Here's how the part is built. I have some questions about the finished solid (model axes, mm). A direction names the side the tool comes from. Round coordinates to 2 decimals unless told otherwise and drop trailing zeros. Write each loop counter-clockwise with the first axis right and the second up, starting at its lowest first coordinate (ties: lowest second). Pieces come first, ordered by that corner, then holes. Notation, with made-up numbers: (-39, 66.25) -> (13, 66.25) arc R19 ccw to (13, 99.25) -> close; hole circle Ø1 at (65, -1). An arc over 180 degrees is marked (long way). Put each result on its own line as item: value. Start each with the question number.
1. I need wall thicknesses on probe 1 along Z at (x, y) = (-10, -12); probe 2 along X at (y, z) = (-15, 22); probe 3 along X at (y, z) = (-8.5, -10.5). Which ranges of each line are inside material? Lowest first, please. Write a range as from..to.
2. Which directions (+Z, -Z, +X, -X, +Y, -Y) give clear straight access to the entire face, cutting with the end or side of a thin tool? Please do faces 4 (the face through (81.15, -2, 0)), 5 (the face through (72.57, -15.52, 16.15)), 6 (the face through (48, -17, 0)).
3. We'd pull the mould along Z, two halves only. Please class faces 1 (the face through (0.106, 2.465, -18.398)), 2 (the face through (105, -12, 0)), 3 (the face through (47.474, -15.521, 15.891)): +Z half, -Z half, draft (parallel to the pull), parting line (faces both ways), or undercut.
4. Suppose I cut it at A-A (z = 0). Count the separate pieces of the cut face and the enclosed holes in it, then the cut area to 3 significant figures.
5. Suppose I cut it at C-C (x = 0). Please give me the cut outline in (y, z).
6. For pin 1 (7 mm diameter, centred on x = 62, y = -5.5, fed in from +Z); pin 2 (4 mm diameter, centred on y = 0.5, z = -6, fed in from +X); pin 3 (5 mm diameter, centred on x = 74.5, z = -15.5, fed in from -Y); pin 4 (5 mm diameter, centred on x = 20.86, z = -20.86, fed in from +Y), each with a flat end and sliding along its axis, tell me the tip position at first contact or that it passes through.
7. Suppose I cut it at D-D (x = 75.5). Please give me the cut outline in (y, z).
```python
from build123d import *

# Parameters (mm, degrees)
SKETCH_1_R                   = 38
SKETCH_1_R_2                 = 12
SKETCH_1_R_3                 = 2.4
SKETCH_1_R_4                 = 3.1
EXTRUDE_1_DEPTH              = 5
SKETCH_2_R                   = 8.5
EXTRUDE_2_DEPTH              = 17
SKETCH_3_R                   = 6
CUT_EXTRUDE_1_DEPTH          = 19
CUT_EXTRUDE_2_REACH          = 59
SKETCH_4_R                   = 3.1
CUT_EXTRUDE_START            = 6
CUT_EXTRUDE_3_DEPTH          = 6
EXTRUDE_START                = -22
EXTRUDE_5_DEPTH              = 22
SKETCH_9_W                   = 41.71930009
SKETCH_9_H                   = 2.5
EXTRUDE_6_DEPTH              = 17
CUT_EXTRUDE_4_REACH          = 122.848
SKETCH_10_W                  = 15
SKETCH_10_H                  = 11
SKETCH_11_W                  = 42.3
SKETCH_11_H                  = 42.3
SKETCH_11_R                  = 11.25
CUT_EXTRUDE_5_DEPTH          = 14
CUT_EXTRUDE_6_REACH          = 113.225
SKETCH_11_2_R                = 1.75
SKETCH_11_2_R_2              = 11.25
CHAMFER_2_SIZE               = 4
HOLE_WIZARD_M5_2_D           = 5.5
HOLE_WIZARD_M5_2_CBORE_D     = 11
HOLE_WIZARD_M5_2_CBORE_DEPTH = 0.5
SKETCH_13_R                  = 3
CUT_EXTRUDE_7_DEPTH          = 3


# Read off the part's stored shape, not the designer's step: 凸台-拉伸5
with BuildPart() as part:
    # 草图1 → 凸台-拉伸1 (new body)
    with BuildSketch(Plane(origin=(0, 0, 0), x_dir=(1, 0, 0), z_dir=(0, 1, 0))):
        with Locations(Location((0, 0, 0), (0, 0, 270))):
            Circle(SKETCH_1_R)
        with Locations(Location((0, 0, 0), (0, 0, 270))):
            Circle(SKETCH_1_R_2, mode=Mode.SUBTRACT)
        with Locations(Location((-11.313708499, 11.313708499, 0), (0, 0, 270))):
            Circle(SKETCH_1_R_3, mode=Mode.SUBTRACT)
        with Locations(Location((0, 16, 0), (0, 0, 270))):
            Circle(SKETCH_1_R_3, mode=Mode.SUBTRACT)
        with Locations(Location((11.313708499, 11.313708499, 0), (0, 0, 270))):
            Circle(SKETCH_1_R_3, mode=Mode.SUBTRACT)
        with Locations(Location((11.313708499, -11.313708499, 0), (0, 0, 90))):
            Circle(SKETCH_1_R_3, mode=Mode.SUBTRACT)
        with Locations(Location((-11.313708499, -11.313708499, 0), (0, 0, 90))):
            Circle(SKETCH_1_R_3, mode=Mode.SUBTRACT)
        with Locations(Location((0, -16, 0), (0, 0, 90))):
            Circle(SKETCH_1_R_3, mode=Mode.SUBTRACT)
        with Locations(Location((-20.859650045, 20.859650045, 0), (0, 0, 270))):
            Circle(SKETCH_1_R_4, mode=Mode.SUBTRACT)
        with Locations(Location((20.859650045, 20.859650045, 0), (0, 0, 270))):
            Circle(SKETCH_1_R_4, mode=Mode.SUBTRACT)
        with Locations(Location((20.859650045, -20.859650045, 0), (0, 0, 270))):
            Circle(SKETCH_1_R_4, mode=Mode.SUBTRACT)
        with Locations(Location((-20.859650045, -20.859650045, 0), (0, 0, 270))):
            Circle(SKETCH_1_R_4, mode=Mode.SUBTRACT)
    extrude(amount=EXTRUDE_1_DEPTH)

    # 草图2 → 凸台-拉伸2 (add)
    with BuildSketch(Plane(origin=(0, 0, 0), x_dir=(1, 0, 0), z_dir=(0, 1, 0))):
        with Locations(Location((-20.859650045, 20.859650045, 0), (0, 0, 270))):
            Circle(SKETCH_2_R)
        with Locations(Location((20.859650045, 20.859650045, 0), (0, 0, 270))):
            Circle(SKETCH_2_R)
        with Locations(Location((20.859650045, -20.859650045, 0), (0, 0, 270))):
            Circle(SKETCH_2_R)
        with Locations(Location((-20.859650045, -20.859650045, 0), (0, 0, 270))):
            Circle(SKETCH_2_R)
    extrude(amount=-EXTRUDE_2_DEPTH)

    # 草图3 → 切除-拉伸1 (cut)
    with BuildSketch(Plane(origin=(0, 5, 0), x_dir=(1, 0, 0), z_dir=(0, 1, 0))):
        with Locations(Location((-20.859650045, 20.859650045, 0), (0, 0, 270))):
            Circle(SKETCH_3_R)
        with Locations(Location((20.859650045, 20.859650045, 0), (0, 0, 270))):
            Circle(SKETCH_3_R)
        with Locations(Location((20.859650045, -20.859650045, 0), (0, 0, 270))):
            Circle(SKETCH_3_R)
        with Locations(Location((-20.859650045, -20.859650045, 0), (0, 0, 270))):
            Circle(SKETCH_3_R)
    extrude(amount=-CUT_EXTRUDE_1_DEPTH, mode=Mode.SUBTRACT)

    # 草图4 → 切除-拉伸2 (cut, up to next)
    with BuildSketch(Plane(origin=(0, -14, 0), x_dir=(1, 0, 0), z_dir=(0, 1, 0)), mode=Mode.PRIVATE) as cut_extrude_2_sk1:
        with Locations(Location((-20.859650045, 20.859650045, 0), (0, 0, 270))):
            Circle(SKETCH_4_R)
    cut_extrude_2_tool1 = extrude(cut_extrude_2_sk1.sketch, amount=-CUT_EXTRUDE_2_REACH, mode=Mode.PRIVATE) & part.part
    # 草图4 → 切除-拉伸2 (cut, up to next)
    with BuildSketch(Plane(origin=(0, -14, 0), x_dir=(1, 0, 0), z_dir=(0, 1, 0)), mode=Mode.PRIVATE) as cut_extrude_2_sk2:
        with Locations(Location((20.859650045, 20.859650045, 0), (0, 0, 270))):
            Circle(SKETCH_4_R)
    cut_extrude_2_tool2 = extrude(cut_extrude_2_sk2.sketch, amount=-CUT_EXTRUDE_2_REACH, mode=Mode.PRIVATE) & part.part
    # 草图4 → 切除-拉伸2 (cut, up to next)
    with BuildSketch(Plane(origin=(0, -14, 0), x_dir=(1, 0, 0), z_dir=(0, 1, 0)), mode=Mode.PRIVATE) as cut_extrude_2_sk3:
        with Locations(Location((20.859650045, -20.859650045, 0), (0, 0, 270))):
            Circle(SKETCH_4_R)
    cut_extrude_2_tool3 = extrude(cut_extrude_2_sk3.sketch, amount=-CUT_EXTRUDE_2_REACH, mode=Mode.PRIVATE) & part.part
    # 草图4 → 切除-拉伸2 (cut, up to next)
    with BuildSketch(Plane(origin=(0, -14, 0), x_dir=(1, 0, 0), z_dir=(0, 1, 0)), mode=Mode.PRIVATE) as cut_extrude_2_sk4:
        with Locations(Location((-20.859650045, -20.859650045, 0), (0, 0, 270))):
            Circle(SKETCH_4_R)
    cut_extrude_2_tool4 = extrude(cut_extrude_2_sk4.sketch, amount=-CUT_EXTRUDE_2_REACH, mode=Mode.PRIVATE) & part.part
    add(cut_extrude_2_tool1.solids().sort_by_distance((-20.85965, -14, -20.85965))[0], mode=Mode.SUBTRACT)
    add(cut_extrude_2_tool2.solids().sort_by_distance((20.85965, -14, -20.85965))[0], mode=Mode.SUBTRACT)
    add(cut_extrude_2_tool3.solids().sort_by_distance((20.85965, -14, 20.85965))[0], mode=Mode.SUBTRACT)
    add(cut_extrude_2_tool4.solids().sort_by_distance((-20.85965, -14, 20.85965))[0], mode=Mode.SUBTRACT)

    # 草图7 → 切除-拉伸3 (cut)
    with BuildSketch(Plane(origin=(0, 0, 0), x_dir=(1, 0, 0), z_dir=(0, 1, 0)).offset(CUT_EXTRUDE_START)):
        with BuildLine():
            Line((-20.859650045, -29.359650045), (20.859650045, -29.359650045))
            ThreePointArc((20.859650045, -29.359650045), (24.11245922, -28.712626071), (26.870057685, -26.870057685))
            ThreePointArc((26.870057685, -26.870057685), (0, -38), (-26.870057685, -26.870057685))
            ThreePointArc((-26.870057685, -26.870057685), (-24.11245922, -28.712626071), (-20.859650045, -29.359650045))
        make_face()
        with BuildLine():
            Line((-20.859650045, 29.359650045), (20.859650045, 29.359650045))
            ThreePointArc((20.859650045, 29.359650045), (24.11245922, 28.712626071), (26.870057685, 26.870057685))
            ThreePointArc((26.870057685, 26.870057685), (0, 38), (-26.870057685, 26.870057685))
            ThreePointArc((-26.870057685, 26.870057685), (-24.11245922, 28.712626071), (-20.859650045, 29.359650045))
        make_face()
    extrude(amount=-CUT_EXTRUDE_3_DEPTH, mode=Mode.SUBTRACT)

    # 凸台-拉伸5 outline → 凸台-拉伸5 (add)
    with BuildSketch(Plane(origin=(0, 5, 0), x_dir=(1, 0, 0), z_dir=(0, 1, 0)).offset(EXTRUDE_START)):
        with BuildLine():
            ThreePointArc((-26.870057685, 26.870057685), (-38, 0), (-26.870057685, -26.870057685))
            ThreePointArc((-26.870057685, -26.870057685), (-28.864243736, -23.719104512), (-29.317860266, -20.017818797))
            ThreePointArc((-29.317860266, -20.017818797), (-35.5, 0), (-29.317860266, 20.017818797))
            ThreePointArc((-29.317860266, 20.017818797), (-28.864243736, 23.719104512), (-26.870057685, 26.870057685))
        make_face()
        with BuildLine():
            ThreePointArc((28.135986341, 16.465912444), (32.6, 0), (28.135986341, -16.465912444))
            ThreePointArc((28.135986341, -16.465912444), (28.333920326, -24.907524026), (21.155863292, -29.354487166))
            Line((21.155863292, -29.354487166), (60, -28))
            Line((60, -28), (105, -28))
            Line((105, -28), (105, 28))
            Line((105, 28), (60, 28))
            Line((60, 28), (21.155863292, 29.354487166))
            ThreePointArc((21.155863292, 29.354487166), (28.333920326, 24.907524026), (28.135986341, 16.465912444))
        make_face()
    extrude(amount=EXTRUDE_5_DEPTH)

    # 草图9 → 凸台-拉伸6 (add)
    with BuildSketch(Plane.XZ):
        with Locations((0, 28.109650045)):
            Rectangle(SKETCH_9_W, SKETCH_9_H)
        with Locations((0, -28.109650045)):
            Rectangle(SKETCH_9_W, SKETCH_9_H)
    extrude(amount=EXTRUDE_6_DEPTH)

    # 草图10 → 切除-拉伸4 (cut, up to next)
    with BuildSketch(Plane.XY.offset(28), mode=Mode.PRIVATE) as cut_extrude_4_sk1:
        with Locations((97.5, -0.5)):
            Rectangle(SKETCH_10_W, SKETCH_10_H)
    cut_extrude_4_tool1 = extrude(cut_extrude_4_sk1.sketch, amount=-CUT_EXTRUDE_4_REACH, mode=Mode.PRIVATE) & part.part
    add(cut_extrude_4_tool1.solids().sort_by_distance((97.5, -0.5, 28))[0], mode=Mode.SUBTRACT)

    # 草图11 → 切除-拉伸5 (cut)
    with BuildSketch(Plane(origin=(0, 5, 0), x_dir=(1, 0, 0), z_dir=(0, 1, 0))):
        with Locations((60, 0)):
            Rectangle(SKETCH_11_W, SKETCH_11_H)
        with Locations(Location((60, 0, 0), (0, 0, 270))):
            Circle(SKETCH_11_R, mode=Mode.SUBTRACT)
    extrude(amount=-CUT_EXTRUDE_5_DEPTH, mode=Mode.SUBTRACT)

    # 草图11<2> → 切除-拉伸6 (cut, up to next)
    with BuildSketch(Plane(origin=(0, 5, 0), x_dir=(1, 0, 0), z_dir=(0, 1, 0)), mode=Mode.PRIVATE) as cut_extrude_6_sk1:
        with Locations(Location((44.5, 15.5, 0), (0, 0, 270))):
            Circle(SKETCH_11_2_R)
    cut_extrude_6_tool1 = extrude(cut_extrude_6_sk1.sketch, amount=-CUT_EXTRUDE_6_REACH, mode=Mode.PRIVATE) & part.part
    # 草图11<2> → 切除-拉伸6 (cut, up to next)
    with BuildSketch(Plane(origin=(0, 5, 0), x_dir=(1, 0, 0), z_dir=(0, 1, 0)), mode=Mode.PRIVATE) as cut_extrude_6_sk2:
        with Locations(Location((60, 0, 0), (0, 0, 270))):
            Circle(SKETCH_11_2_R_2)
    cut_extrude_6_tool2 = extrude(cut_extrude_6_sk2.sketch, amount=-CUT_EXTRUDE_6_REACH, mode=Mode.PRIVATE) & part.part
    # 草图11<2> → 切除-拉伸6 (cut, up to next)
    with BuildSketch(Plane(origin=(0, 5, 0), x_dir=(1, 0, 0), z_dir=(0, 1, 0)), mode=Mode.PRIVATE) as cut_extrude_6_sk3:
        with Locations(Location((75.5, 15.5, 0), (0, 0, 270))):
            Circle(SKETCH_11_2_R)
    cut_extrude_6_tool3 = extrude(cut_extrude_6_sk3.sketch, amount=-CUT_EXTRUDE_6_REACH, mode=Mode.PRIVATE) & part.part
    # 草图11<2> → 切除-拉伸6 (cut, up to next)
    with BuildSketch(Plane(origin=(0, 5, 0), x_dir=(1, 0, 0), z_dir=(0, 1, 0)), mode=Mode.PRIVATE) as cut_extrude_6_sk4:
        with Locations(Location((75.5, -15.5, 0), (0, 0, 270))):
            Circle(SKETCH_11_2_R)
    cut_extrude_6_tool4 = extrude(cut_extrude_6_sk4.sketch, amount=-CUT_EXTRUDE_6_REACH, mode=Mode.PRIVATE) & part.part
    # 草图11<2> → 切除-拉伸6 (cut, up to next)
    with BuildSketch(Plane(origin=(0, 5, 0), x_dir=(1, 0, 0), z_dir=(0, 1, 0)), mode=Mode.PRIVATE) as cut_extrude_6_sk5:
        with Locations(Location((44.5, -15.5, 0), (0, 0, 270))):
            Circle(SKETCH_11_2_R)
    cut_extrude_6_tool5 = extrude(cut_extrude_6_sk5.sketch, amount=-CUT_EXTRUDE_6_REACH, mode=Mode.PRIVATE) & part.part
    add(cut_extrude_6_tool1.solids().sort_by_distance((44.5, 5, -15.5))[0], mode=Mode.SUBTRACT)
    add(cut_extrude_6_tool2.solids().sort_by_distance((60, 5, 0))[0], mode=Mode.SUBTRACT)
    add(cut_extrude_6_tool3.solids().sort_by_distance((75.5, 5, -15.5))[0], mode=Mode.SUBTRACT)
    add(cut_extrude_6_tool4.solids().sort_by_distance((75.5, 5, 15.5))[0], mode=Mode.SUBTRACT)
    add(cut_extrude_6_tool5.solids().sort_by_distance((44.5, 5, 15.5))[0], mode=Mode.SUBTRACT)

    # 倒角2
    chamfer_2_edges = [part.edges().sort_by_distance(p)[0] for p in [
        (38.85, -2, -21.15),
        (81.15, -2, -21.15),
        (81.15, -2, 21.15),
        (38.85, -2, 21.15),
    ]]
    chamfer(chamfer_2_edges, length=CHAMFER_2_SIZE)

    # M5 六角头螺栓的柱形沉头孔2 (through all)
    with Locations(Plane(origin=(0, -17, 0), x_dir=(-1, 0, 0), z_dir=(0, -1, 0))):
        with Locations((-97.5, -16), (-97.5, 0), (-97.5, 16)):
            CounterBoreHole(HOLE_WIZARD_M5_2_D / 2, HOLE_WIZARD_M5_2_CBORE_D / 2, HOLE_WIZARD_M5_2_CBORE_DEPTH)

    # 草图13 → 切除-拉伸7 (cut)
    with BuildSketch(Plane.XZ.offset(17)):
        with Locations(Location((44.5, 15.5, 0), (0, 0, 270))):
            Circle(SKETCH_13_R)
        with Locations(Location((75.5, 15.5, 0), (0, 0, 270))):
            Circle(SKETCH_13_R)
        with Locations(Location((75.5, -15.5, 0), (0, 0, 270))):
            Circle(SKETCH_13_R)
        with Locations(Location((44.5, -15.5, 0), (0, 0, 270))):
            Circle(SKETCH_13_R)
    extrude(amount=-CUT_EXTRUDE_7_DEPTH, mode=Mode.SUBTRACT)


solid = part.part
```
Verdict:
1. probe 1: z = -29.36..-26.86, 26.86..29.36
1. probe 2: x = -30.98..-23.74, -17.98..-12.44, 12.44..17.98, 23.74..105
1. probe 3: x = -36.52..-33.91, 30.86..38.85, 81.15..105
2. face 4: +Y
2. face 5: -Y
2. face 6: +Z, -Z, +X, -X, -Y
3. face 1: undercut
3. face 2: draft
3. face 3: undercut
4. separate pieces: 4
4. enclosed holes: 0
4. area: 868 mm^2
5. outline: (-17, -29.36) -> (5, -29.36) -> (5, -18.4) -> (0, -18.4) -> (0, -26.86) -> (-17, -26.86) -> close; (-17, 26.86) -> (0, 26.86) -> (0, 18.4) -> (5, 18.4) -> (5, 29.36) -> (-17, 29.36) -> close; (0, -13.6) -> (5, -13.6) -> (5, -12) -> (0, -12) -> close; (0, 12) -> (5, 12) -> (5, 13.6) -> (0, 13.6) -> close
6. pin 1: stops at z = 28.05
6. pin 2: stops at x = 90
6. pin 3: stops at y = -17
6. pin 4: passes through
7. outline: (-17, -28) -> (5, -28) -> (5, -21.15) -> (-9, -21.15) -> (-9, -17.25) -> (-14, -17.25) -> (-14, -18.5) -> (-17, -18.5) -> close; (-17, -12.5) -> (-14, -12.5) -> (-14, -13.75) -> (-9, -13.75) -> (-9, 13.75) -> (-14, 13.75) -> (-14, 12.5) -> (-17, 12.5) -> close; (-17, 18.5) -> (-14, 18.5) -> (-14, 17.25) -> (-9, 17.25) -> (-9, 21.15) -> (5, 21.15) -> (5, 28) -> (-17, 28) -> close
